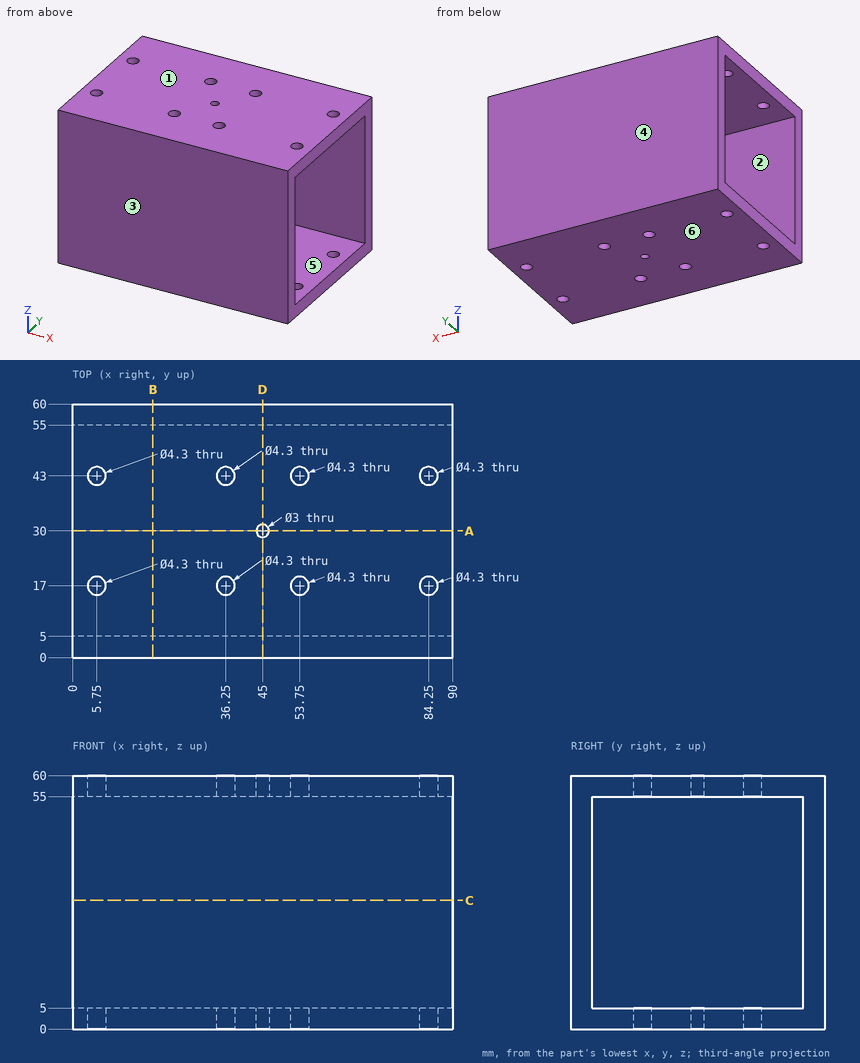
Geometry check sheet. Reference: drawing and pictorial views, mm from the part's lowest x, y, z. A direction names the side the tool comes from. Give positions to 0.01 mm unless a question says otherwise; leave off trailing zeros. Order: outer loops, then holes, each group sorted by start corner. A loop starts at its lowest first (then second) coordinate and runs counter-clockwise, first axis right, second up. Notation, with made-up numbers: (75.25, 73.25) -> (86.25, 73.25) arc R32 ccw to (86.25, 107.25) -> close; hole circle Ø3 at (-5, 34.25). An arc over 180 degrees is marked (long way). Write each question's results on one line, items separated by ' | '. Start each with the question number.
(1) Sectioned sample at C-C (z = 30.5). Enter the section's corners in (x, y).
(2) Sectioned sample at B-B (x = 19). Enter the section's corners in (y, z), plus the area to 3 significant figures.
(3) Scan lines: line 1 (Y direction, x = 5.75, z = 1.75); line 2 (Y direction, x = 45, z = 1.75); line 3 (Z direction, x = 86, y = 15). Record each from-to range of solid material in increasing order.
(4) Sectioned sample at A-A (y = 30). Enter the section's corners in (x, z).
(5) Mould release check, pull along Y, two halves, no side actions. Record for the marked faces 1, 2, 3 and 4: pulls with the +Y half, pulls with the -Y half, needs draft (parallel to the pull), parting line crosses it, or undercut.
(6) Access from +Z, -Z, +X, -X, +Y, -Y to the whole of each face (thin tool, end or side, straight path). Record for the marked faces 5 and 6.
(7) Sectioned sample at D-D (x = 45). Enter the section's corners in (y, z), plus the area to 3 significant figures.
Answer below:
1) outline: (0, 0) -> (90, 0) -> (90, 5) -> (0, 5) -> close; (0, 55) -> (90, 55) -> (90, 60) -> (0, 60) -> close
2) outline: (0, 0) -> (60, 0) -> (60, 60) -> (0, 60) -> close; hole (5, 5) -> (55, 5) -> (55, 55) -> (5, 55) -> close | area: 1,100 mm2
3) line 1: 0 to 14.85, 19.15 to 40.85, 45.15 to 60 | line 2: 0 to 28.5, 31.5 to 60 | line 3: 0 to 5, 55 to 60
4) outline: (0, 0) -> (43.5, 0) -> (43.5, 5) -> (0, 5) -> close; (0, 55) -> (43.5, 55) -> (43.5, 60) -> (0, 60) -> close; (46.5, 0) -> (90, 0) -> (90, 5) -> (46.5, 5) -> close; (46.5, 55) -> (90, 55) -> (90, 60) -> (46.5, 60) -> close
5) face 1: needs draft | face 2: undercut | face 3: pulls with the -Y half | face 4: pulls with the +Y half
6) face 5: +X, -X | face 6: -Z, +X, -X, +Y, -Y
7) outline: (0, 0) -> (28.5, 0) -> (28.5, 5) -> (5, 5) -> (5, 55) -> (28.5, 55) -> (28.5, 60) -> (0, 60) -> close; (31.5, 0) -> (60, 0) -> (60, 60) -> (31.5, 60) -> (31.5, 55) -> (55, 55) -> (55, 5) -> (31.5, 5) -> close | area: 1,070 mm2
